```python
from build123d import *

# Parameters (mm, degrees)
SKETCH2_R               = 15.5
BOSS_EXTRUDE1_DEPTH     = 30
FILLET1_R               = 3
CUT_EXTRUDE1_DEPTH      = 20
CUT_EXTRUDE1_DEPTH_BACK = 20


with BuildPart() as part:
    # Sketch2 → Boss-Extrude1 (new body)
    with BuildSketch(Plane.XY):
        Circle(SKETCH2_R)
    extrude(amount=BOSS_EXTRUDE1_DEPTH)

    # Fillet1
    fillet1_edges = [part.edges().sort_by_distance(p)[0] for p in [
        (-15.5, 0, 0),
        (-15.5, 0, 30),
    ]]
    fillet(fillet1_edges, radius=FILLET1_R)

    # Sketch3 → Cut-Extrude1 (cut, two sides: drawn at the far end of the back side and taken through both)
    with BuildSketch(Plane(origin=(0, 0, 0), x_dir=(1, 0, 0), z_dir=(0, 1, 0)).offset(-CUT_EXTRUDE1_DEPTH_BACK)):
        with BuildLine():
            Line((4.854198749, 0), (19.206398093, 0))
            Line((19.206398093, 0), (19.206398093, -15.636699312))
            Line((19.206398093, -15.636699312), (15.5, -15.636699312))
            add(Edge.make_bspline(
                [(4.854198749, 0), (12.000659595, -6.632087606), (15.5, -15.636699312)],
                knots=[0, 0, 0, 1, 1, 1], degree=2))
        make_face()
    extrude(amount=CUT_EXTRUDE1_DEPTH + CUT_EXTRUDE1_DEPTH_BACK, mode=Mode.SUBTRACT)


solid = part.part
```
Can you work these out from the model? Positions are in its coordinate system, mm. Round coordinates to 2 decimals unless told otherwise and drop trailing zeros. Order: outer loops, then holes, each group sorted by start corner. A loop starts at its lowest first (then second) coordinate and runs counter-clockwise, first axis right, second up.
(1) If we section it at B-B (z = 28): Please give me the cut outline in (x, y), plus the area to 3 significant figures.
Results are:
outline: circle Ø30.66 at (0, 0)
area: 738 mm2
(2) I'm going to push flat-ended pins straight in: pin 1 (2 mm diameter, centred on x = -11.5, y = -8.5, fed in from -Z); pin 2 (4 mm diameter, centred on x = -9, z = 5.5, fed in from -Y); pin 3 (2 mm diameter, centred on y = -9.5, z = 17, fed in from +X); pin 4 (2 mm diameter, centred on x = -0.5, z = 6.5, fed in from +Y). Where does each tip first touch, or does it pass through?
Results are:
pin 1: stops at z = 0.11
pin 2: stops at y = -13.83
pin 3: stops at x = 12.96
pin 4: stops at y = 15.5
(3) If I drill on L1, parallel to Y at x = 0.5, z = 8; L2, parallel to Z at x = -4, y = 12; L3, parallel to Y at x = -7, z = 2, over which ranges is the centre line in solid material (lowest first)?
Results are:
L1: y = -15.49 to 15.49
L2: z = 0 to 30
L3: y = -13.64 to 13.64
(4) If we section it at A-A (z = 18.5): Please give me the cut outline in (x, y).
Results are:
outline: circle Ø31 at (0, 0)
